Job drawing, mm, ordinate dimensions from the low corner. One solid piece. Give positions to 0.01 mm unless a question says otherwise; leave off trailing zeros. Loops run counter-clockwise (first coordinate to the right, second up) from the corner with the lowest first, then second, coordinate; pieces in that order, holes last. Notation, with made-up numbers: (66, 28) -> (121, 28) arc R16 cw to (121, 48) -> close; hole circle Ø4 at (-36, 45). An arc over 180 degrees is marked (long way). Use one line per item in the form item = value.
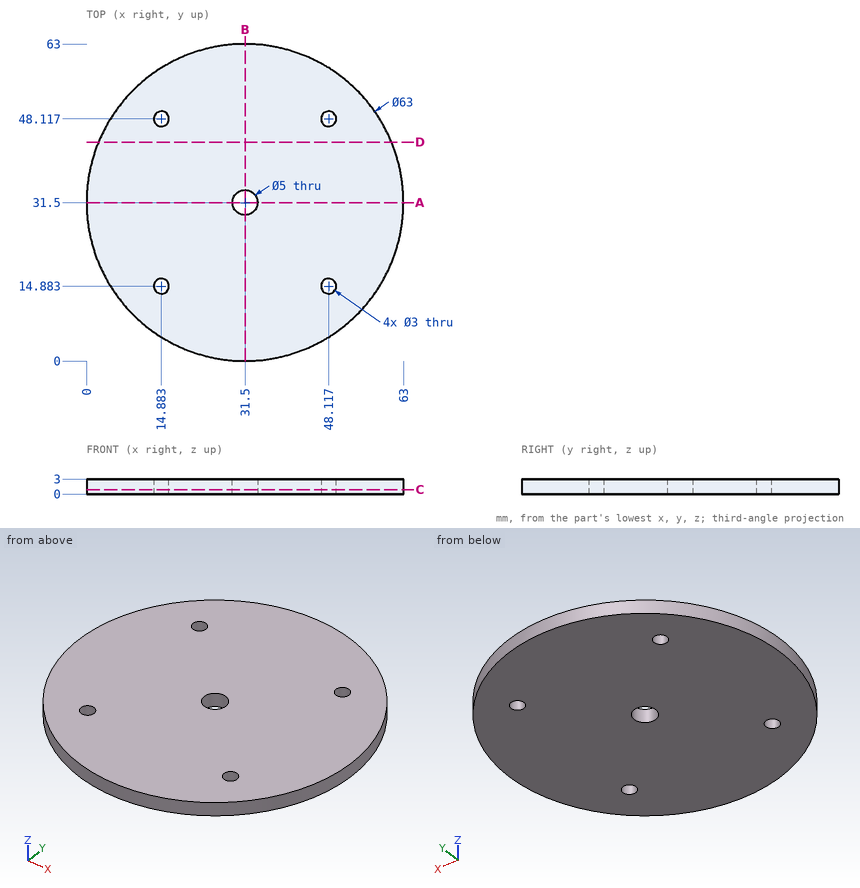
1. Cut at A-A, the plane y = 31.5. Write the cut outline in (x, z), then the cut area to 3 significant figures.
Result sheet:
outline = (0, 0) -> (29, 0) -> (29, 3) -> (0, 3) -> close; (34, 0) -> (63, 0) -> (63, 3) -> (34, 3) -> close
area = 174 mm^2
2. Drop flat-ended pins along their axis: P1, Ø1, axis at y = 50, z = 0.5, coming from the -X side; P2, Ø1.5, axis at x = 46.5, z = 1.5, coming from the -Y side; P3, Ø1.5, axis at y = 23, z = 2.5, coming from the +X side; P4, Ø2.5, axis at x = 14.88, y = 48.12, coming from the -Z side. Give the stop position or say it passes through.
Result sheet:
P1 = 5.65
P2 = 3.41
P3 = 62.03
P4 = through
3. Cut at D-D, the plane y = 43.5. Write the cut outline in (x, z).
Result sheet:
outline = (2.38, 0) -> (60.62, 0) -> (60.62, 3) -> (2.38, 3) -> close
4. Cut at C-C, the plane z = 0.9. Write the cut outline in (x, y).
Result sheet:
outline = circle Ø63 at (31.5, 31.5); hole circle Ø3 at (14.88, 14.88); hole circle Ø3 at (14.88, 48.12); hole circle Ø5 at (31.5, 31.5); hole circle Ø3 at (48.12, 14.88); hole circle Ø3 at (48.12, 48.12)
5. Drill centre lines: line 1 (X direction, y = 33, z = 1); line 2 (X direction, y = 7.5, z = 2.3); line 3 (Y direction, x = 34.5, z = 1.6). Where is each one in solid material? Low to high.
Result sheet:
line_1 = 0.04 to 29.5, 33.5 to 62.96
line_2 = 11.1 to 51.9
line_3 = 0.14 to 62.86
